Source: CAD feature listing. Evaluate the final solid. Frame: model axes, mm. A direction names the side the tool comes from. Round coordinates to 2 decimals unless told otherwise and drop trailing zeros. Loops run counter-clockwise (first coordinate to the right, second up) from the corner with the lowest first, then second, coordinate; pieces in that order, holes last.
(1) Section C-C, the plane x = 7.5. Return the cut outline in (y, z), plus the area to 3 significant figures.
(2) First-contact query: pin 1 Ø1 at (x, y) = (17, 9.5) entering from -Z; pin 2 Ø1.2 at (x, y) = (1.5, 7.5) entering from +Z. Flat tips, straight axial feed; report the tip coordinate or a pass-through.
(3) Set-up query: faces 4 (the flat face through (10, -3.5, 11)), 5 (the flat face through (7, 12, 3)). Return all of +Z, -Z, +X, -X, +Y, -Y with unobstructed straight access to the full face (end or side cutting, diameter ignored); none if empty.
(4) Mould query, pull axis X, two halves, no side actions, for faces 1 (the flat face through (10, 26.5, 11)), 2 (the flat face through (2.4, 12, 12)), 3 (the flat face through (-4.5, 11, 11)). Classes: pulls with the +X half, pulls with the -X half, needs draft (parallel to the pull), parting line crosses it, or undercut.
(5) Section B-B, the plane y = 13.5. Return the cut outline in (x, z), plus the area to 3 significant figures.
(6) Material intervals for probe 1 along X at (y, z) = (1.25, 17.5); probe 2 along Y at (x, z) = (17.5, 16.5); probe 3 along Z at (x, y) = (18.5, 9.5), sorted ascending.
(7) Section A-A, the plane z = 17.25. Return the cut outline in (x, y).
```python
from build123d import *

# Parameters (mm, degrees)
BOX001_W     = 2.4
BOX001_H     = 24
BOX001_DEPTH = 22
BOX002_W     = 2.4
BOX002_H     = 24
BOX002_DEPTH = 22
BOX003_W     = 2.4
BOX003_H     = 24
BOX003_DEPTH = 22
BOX_W        = 2.4
BOX_H        = 24
BOX_DEPTH    = 22
BOX004_W     = 29
BOX004_H     = 30
BOX004_DEPTH = 22


with BuildPart() as ranura2:
    # Box001 → Box001 (new body)
    with BuildSketch(Plane(origin=(5.6, 0, 0), x_dir=(1, 0, 0), z_dir=(0, 0, 1))):
        with Locations((1.2, 12)):
            Rectangle(BOX001_W, BOX001_H)
    extrude(amount=BOX001_DEPTH)


with BuildPart() as ranura3:
    # Box002 → Box002 (new body)
    with BuildSketch(Plane(origin=(11.2, 0, 0), x_dir=(1, 0, 0), z_dir=(0, 0, 1))):
        with Locations((1.2, 12)):
            Rectangle(BOX002_W, BOX002_H)
    extrude(amount=BOX002_DEPTH)


with BuildPart() as ranura4:
    # Box003 → Box003 (new body)
    with BuildSketch(Plane(origin=(16.8, 0, 0), x_dir=(1, 0, 0), z_dir=(0, 0, 1))):
        with Locations((1.2, 12)):
            Rectangle(BOX003_W, BOX003_H)
    extrude(amount=BOX003_DEPTH)


with BuildPart() as ranuras:
    # Box → Box (new body)
    with BuildSketch(Plane.XY):
        with Locations((1.2, 12)):
            Rectangle(BOX_W, BOX_H)
    extrude(amount=BOX_DEPTH)

    # Fusion: union ranura2, ranura3, ranura4
    add(ranura2.part)
    add(ranura3.part)
    add(ranura4.part)


with BuildPart() as ranuras_1:
    # Fusion placement: moved
    add(ranuras.part.moved(Location((0, 0, 3))))


with BuildPart() as cut:
    # Box004 → Box004 (new body)
    with BuildSketch(Plane(origin=(-4.5, -3.5, 0), x_dir=(1, 0, 0), z_dir=(0, 0, 1))):
        with Locations((14.5, 15)):
            Rectangle(BOX004_W, BOX004_H)
    extrude(amount=BOX004_DEPTH)

    # Cut: cut ranuras
    add(ranuras_1.part, mode=Mode.SUBTRACT)


solid = cut.part
```
Output values:
1. outline: (-3.5, 0) - (26.5, 0) - (26.5, 22) - (24, 22) - (24, 3) - (0, 3) - (0, 22) - (-3.5, 22) - close
1. area: 204 mm2
2. pin 1: stops at z = 0
2. pin 2: stops at z = 3
3. face 4: +Z, -Z, +X, -X, -Y
3. face 5: +Z
4. face 1: needs draft
4. face 2: undercut
4. face 3: pulls with the -X half
5. outline: (-4.5, 0) - (24.5, 0) - (24.5, 22) - (19.2, 22) - (19.2, 3) - (16.8, 3) - (16.8, 22) - (13.6, 22) - (13.6, 3) - (11.2, 3) - (11.2, 22) - (8, 22) - (8, 3) - (5.6, 3) - (5.6, 22) - (2.4, 22) - (2.4, 3) - (0, 3) - (0, 22) - (-4.5, 22) - close
5. area: 456 mm2
6. probe 1: x = -4.5 to 0, 2.4 to 5.6, 8 to 11.2, 13.6 to 16.8, 19.2 to 24.5
6. probe 2: y = -3.5 to 0, 24 to 26.5
6. probe 3: z = 0 to 3
7. outline: (-4.5, -3.5) - (24.5, -3.5) - (24.5, 26.5) - (-4.5, 26.5) - close; hole (0, 0) - (2.4, 0) - (2.4, 24) - (0, 24) - close; hole (5.6, 0) - (8, 0) - (8, 24) - (5.6, 24) - close; hole (11.2, 0) - (13.6, 0) - (13.6, 24) - (11.2, 24) - close; hole (16.8, 0) - (19.2, 0) - (19.2, 24) - (16.8, 24) - close
